For this review, take the finished solid that the model builds, in its own axes (mm). A direction names the side the tool comes from. Round coordinates to 2 decimals unless told otherwise and drop trailing zeros. Write each loop counter-clockwise with the first axis right and the second up, starting at its lowest first coordinate (ties: lowest second). Pieces come first, ordered by that corner, then holes. Notation, with made-up numbers: M 27,64.5 L 70,64.5 A17 ccw 70,91.5 Z; hole C -25,-25.5 d1. An arc over 180 degrees is marked long. Answer in a Markdown table with one row per item.
```python
from build123d import *

# Parameters (mm, degrees)
SKETCH1_W           = 60
SKETCH1_H           = 5
BOSS_EXTRUDE1_DEPTH = 10
SKETCH2_W           = 4
SKETCH2_H           = 10
FILLET1_R           = 2


with BuildPart() as part:
    # Sketch1 → Boss-Extrude1 (new body)
    with BuildSketch(Plane(origin=(0, 0, 0), x_dir=(1, 0, 0), z_dir=(0, 1, 0))):
        Rectangle(SKETCH1_W, SKETCH1_H)
    extrude(amount=BOSS_EXTRUDE1_DEPTH)

    # Sweep6: sweep along a curve in space
    with BuildLine() as sweep6_path:
        Line((-25, 5, 2.5), (-25, 5, 9.5))
        ThreePointArc((-25, 5, 9.5), (-22.656854249, 5, 15.156854249), (-17, 5, 17.5))
        Line((-17, 5, 17.5), (17, 5, 17.5))
        ThreePointArc((17, 5, 17.5), (22.656854249, 5, 15.156854249), (25, 5, 9.5))
        Line((25, 5, 2.5), (25, 5, 9.5))
    # Sketch2 → Sweep6 (sweep)
    with BuildSketch(Plane.XY.offset(2.5)):
        with Locations((-25, 5)):
            Rectangle(SKETCH2_W, SKETCH2_H)
    sweep(path=sweep6_path.line)

    # Fillet1
    fillet1_edges = [part.edges().sort_by_distance(p)[0] for p in [
        (-21.242640687, 0, 13.742640687),
        (0, 0, 15.5),
        (21.242640687, 0, 13.742640687),
        (-24.071067812, 0, 16.571067812),
        (0, 0, 19.5),
        (24.071067812, 0, 16.571067812),
        (-28.5, 0, 2.5),
        (-27, 0, 6),
        (-27, 10, 6),
        (-23, 0, 6),
        (0, 0, 2.5),
        (23, 0, 6),
        (27, 0, 6),
        (27, 10, 6),
        (28.5, 0, 2.5),
        (30, 0, 0),
        (0, 0, -2.5),
        (-30, 0, 0),
        (-24.071067812, 10, 16.571067812),
        (24.071067812, 10, 16.571067812),
        (-21.242640687, 10, 13.742640687),
        (21.242640687, 10, 13.742640687),
        (-30, 5, -2.5),
        (-30, 5, 2.5),
        (30, 5, 2.5),
        (30, 5, -2.5),
        (0, 10, -2.5),
        (30, 10, 0),
        (28.5, 10, 2.5),
        (23, 10, 6),
        (0, 10, 2.5),
        (-23, 10, 6),
        (-28.5, 10, 2.5),
        (-30, 10, 0),
        (0, 10, 19.5),
        (0, 10, 15.5),
    ]]
    fillet(fillet1_edges, radius=FILLET1_R - 0.0001)  # a hair under: the kernel refuses the full size


solid = part.part
```
Q1. Mouldability with a two-part tool opening along Z and no side actions: class faces 1 (the face through (0.39, 0.6, -1.93)), 2 (the face through (-29.43, 5.04, 1.9)), 3 (the face through (-21.289, 5.042, 13.696)) as +Z half, -Z half, draft (parallel to the pull), parting line (faces both ways), or undercut.
Found:
| item | result |
|---|---|
| face 1 | -Z half |
| face 2 | +Z half |
| face 3 | undercut |
Q2. Machinability: for faces 4 (the face through (0.24, 0.57, 16.1)), 5 (the face through (-26.4, 9.43, 6.06)), 6 (the face through (-27.1, 0.4, 1.7)), 7 (the face through (0.24, 9.43, 16.1)), which of the approach directions +Z, -Z, +X, -X, +Y, -Y give a long, thin tool a straight path to every point of the face, cutting with its end or side? Answer none if there is none.
Found:
| item | result |
|---|---|
| face 4 | -Y |
| face 5 | +Z, -X, +Y |
| face 6 | +Z, -X, -Y |
| face 7 | +Y |
Q3. Insertion check: P1, Ø3, axis at y = 4, z = 7.5, coming from the +X side; P2, Ø5, axis at y = 5, z = 5.5, coming from the -X side; P3, Ø0.5, axis at x = 27.5, y = 5.5, coming from the +Z side; P4, Ø6, axis at x = -18, y = 5, coming from the +Z side. Each pin has a flat end and moves straight along its axis. Give the tip position at first contact, or say it passes through.
Found:
| item | result |
|---|---|
| P1 | x = 27 |
| P2 | x = -27 |
| P3 | z = 2.5 |
| P4 | z = 19.5 |
Q4. Take a section at C-C (y = 5). State the section outline as (x, z) points, then the cut area to 3 significant figures.
Found:
| item | result |
|---|---|
| outline | M -30,-0.5 A2 ccw -28,-2.5 L 28,-2.5 A2 ccw 30,-0.5 L 30,0.5 A2 ccw 28,2.5 L 27,2.5 L 27,9.5 A10 ccw 17,19.5 L -17,19.5 A10 ccw -27,9.5 L -27,2.5 L -28,2.5 A2 ccw -30,0.5 Z; hole M -23,2.5 L 23,2.5 L 23,9.5 A6 ccw 17,15.5 L -17,15.5 A6 ccw -23,9.5 Z |
| area | 589 mm² |
Q5. For probe 1 along Z at (x, y) = (-0.5, 5); probe 2 along X at (y, z) = (4, 9); probe 3 along X at (y, z) = (5.75, 11), list the stretches that pass through material, from the lowest coordinate up.
Found:
| item | result |
|---|---|
| probe 1 | -2.5 to 2.5, 15.5 to 19.5 |
| probe 2 | -27 to -23, 23 to 27 |
| probe 3 | -26.89 to -22.81, 22.81 to 26.89 |
Q6. Take a section at D-D (y = 1). State the section outline as (x, z) points, then the cut area to 3 significant figures.
Found:
| item | result |
|---|---|
| outline | M -29.73,-0.5 A1.73 ccw -28,-2.23 L 28,-2.23 A1.73 ccw 29.73,-0.5 L 29.73,0.5 A1.73 ccw 28,2.23 L 26.73,2.23 L 26.73,9.5 A9.73 ccw 17,19.23 L -17,19.23 A9.73 ccw -26.73,9.5 L -26.73,2.23 L -28,2.23 A1.73 ccw -29.73,0.5 Z; hole M -23.27,2.23 L 23.27,2.23 L 23.27,9.5 A6.27 ccw 17,15.77 L -17,15.77 A6.27 ccw -23.27,9.5 Z |
| area | 518 mm² |
